```python
from build123d import *

# Parameters (mm, degrees)
FILLET1_R       = 1.5
SKETCH3_W       = 1.42
SKETCH3_H       = 6.6
SKETCH4_W       = 1.42
SKETCH4_H       = 3.159787024
RECPAT_COUNT    = 2
RECPAT_ANGLE    = 90
THDSCHPAT_COUNT = 39
THDSCHPAT_PITCH = 1


with BuildPart() as part:
    # BodySke → Base-Revolve (revolve)
    with BuildSketch(Plane.XY, mode=Mode.PRIVATE) as base_revolve_sk:
        Polygon((0, 0), (0, 5.65), (0.65, 5.65), (3.3, 3), (50, 3), (50, 0), align=None)
    revolve(base_revolve_sk.sketch.rotate(Axis((-6.35, 0, 0), (1, 0, 0)), 90), axis=Axis((-6.35, 0, 0), (1, 0, 0)))

    # Fillet1
    fillet1_edges = [part.edges().sort_by_distance(p)[0] for p in [
        (3.3, 0, -3),
    ]]
    fillet(fillet1_edges, radius=FILLET1_R)

    # Sketch3 → Recess section 0
    with BuildSketch(Plane.ZY):
        Rectangle(SKETCH3_W, SKETCH3_H)
    # Sketch4 → Recess section 1
    with BuildSketch(Plane.ZY.offset(-3.45)):
        Rectangle(SKETCH4_W, SKETCH4_H)
    recess = loft(mode=Mode.SUBTRACT)

    # RecPat: Recess ×2 about axis
    recpat_axis = Axis((0, 0, 0), (1, 0, 0))
    for i in range(1, RECPAT_COUNT):
        add(recess.rotate(recpat_axis, i * RECPAT_ANGLE / (RECPAT_COUNT - 1)), mode=Mode.SUBTRACT)

    # RecCorSke → RecessCore (revolve, cut)
    with BuildSketch(Plane.XY, mode=Mode.PRIVATE) as recesscore_sk:
        Polygon((0, 0), (0, 1.521747501), (3.45, 1.2805), (3.866059671, 0), align=None)
    revolve(recesscore_sk.sketch.rotate(Axis((-3.175, 0, 0), (1, 0, 0)), 90), axis=Axis((-3.175, 0, 0), (1, 0, 0)), mode=Mode.SUBTRACT)

    # ThdSchSke → ThreadSchematic (revolve, cut)
    with BuildSketch(Plane.XY, mode=Mode.PRIVATE) as threadschematic_sk:
        Polygon((12.000001, -2.4455), (11.61173592, -3), (11.61173592, -3.75), (12.38826608, -3.75), (12.38826608, -3), align=None)
    threadschematic = revolve(threadschematic_sk.sketch.rotate(Axis((-3.175, 0, 0), (1, 0, 0)), 270), axis=Axis((-3.175, 0, 0), (1, 0, 0)), mode=Mode.SUBTRACT)

    # ThdSchPat: ThreadSchematic ×39
    with Locations(*[(i * THDSCHPAT_PITCH, 0, 0) for i in range(1, THDSCHPAT_COUNT)]):
        add(threadschematic, mode=Mode.SUBTRACT)


solid = part.part
```
Can you work these out from the model? Positions are in its coordinate system, mm. Coordinates: 2 decimals unless noted, no trailing zeros. Loops run counter-clockwise (first coordinate to the right, second up) from the corner with the lowest first, then second, coordinate; pieces in that order, holes last.
1) I need wall thicknesses on probe 1 along Z at (x, y) = (38.5, 1.75); probe 2 along Y at (x, z) = (4.5, 0); probe 3 along X at (y, z) = (-2.25, -3.25). Which ranges of each line are inside material? Lowest first, please.
2) Imagine slicing it at A-A on x = 7.5. List the corners of the cut face in (y, z) for me, plus the area to 3 significant figures.
3) For pin 1 (6 mm diameter, centred on x = 22.5, y = -2.5, fed in from +Z); pin 2 (2 mm diameter, centred on x = 23, z = -3.5, fed in from +Y); pin 3 (2 mm diameter, centred on x = 14, z = 2.5, fed in from -Y), each with a flat end and sliding along its axis, tell me the tip position at first contact or that it passes through.
Completed:
1. probe 1: z = -2.44 to 2.44
1. probe 2: y = -3 to 3
1. probe 3: x = 0 to 2.35
2. outline: circle Ø6 at (0, 0)
2. area: 28.3 mm2
3. pin 1: stops at z = 3
3. pin 2: stops at y = 1.53
3. pin 3: stops at y = -2.55
